from build123d import *

# Parameters (mm, degrees)
F0_R     = 152.4
F0_R_2   = 30.734
F1_DEPTH = 12.954
F2_R     = 165.1
F3_DEPTH = 17.78
F4_R     = 165.1
F5_DEPTH = 17.78
F6_R     = 30.1625
F7_DEPTH = 62.66538


with BuildPart() as f1:
    # F0 (on Top) → F1 (new body)
    with BuildSketch(Plane.XY):
        Circle(F0_R)
        Circle(F0_R_2, mode=Mode.SUBTRACT)
    extrude(amount=F1_DEPTH)

    # F2 (on face) → F3 (join)
    with BuildSketch(Plane(origin=(0, 0, 0), x_dir=(1, 0, 0), z_dir=(0, 0, -1))):
        Circle(F2_R)
    extrude(amount=F3_DEPTH)

    # F4 (on face) → F5 (join)
    with BuildSketch(Plane.XY.offset(12.954)):
        Circle(F4_R)
    extrude(amount=F5_DEPTH)

    # F6 (on face) → F7 (cut)
    with BuildSketch(Plane(origin=(0, 0, -17.78), x_dir=(1, 0, 0), z_dir=(0, 0, -1))):
        Circle(F6_R)
    extrude(amount=-F7_DEPTH, mode=Mode.SUBTRACT)


solid = f1.part
Model file for the job. Use its own axes, mm. A direction names the side the tool comes from. Coordinates: 2 decimals unless noted, no trailing zeros. Write each loop counter-clockwise with the first axis right and the second up, starting at its lowest first coordinate (ties: lowest second). Pieces come first, ordered by that corner, then holes. Notation, with made-up numbers: (-25.75, 12.5) -> (6.25, 12.5) arc R23 cw to (6.25, 37.5) -> close; hole circle Ø3 at (71.5, -17). An arc over 180 degrees is marked (long way). One line per item, written item: value. Start each with the question number.
1) Which spindle directions (+Z, -Z, +X, -X, +Y, -Y) get a long thin tool onto all of the face, cutting with end or side? Do faces 4 (the face through (-35.79, -161.174, 21.72)), 5 (the face through (48, -146, 12.954)). Say none if no direction does.
2) Slice it at D-D on z = 18. Write the cut outline in (x, y) (1 decimal).
3) Probe probe 1 along X at (y, z) = (0, -11.75); probe 2 along Y at (x, z) = (0, 7.75). List the from-to ranges inside material, lowest first.
4) Slice it at C-C on x = 45.5. Write the cut outline in (y, z), then the cut area to 3 significant figures.
5) Pull direction X, two halves, no side cores. Call faces 1 (the face through (48, 146, 0)), 2 (the face through (-120.94, -92.73, 6.39)), 3 (the face through (23, 20, 0)): +X half, -X half, draft (parallel to the pull), parting line (faces both ways), or undercut.
6) Flat gauge pins, fed straight in: pin 1 Ø12 at (y, z) = (-114.5, -11) entering from -X; pin 2 Ø5 at (y, z) = (78.5, 17) entering from -X; pin 3 Ø10 at (y, z) = (-96, 25) entering from +X; pin 4 Ø18.5 at (x, y) = (13.5, 8) entering from +Z. Where does each tip first touch, or does it go through?
7) Slice it at A-A on y = 0. Write the cut outline in (x, z), then the cut area to 3 significant figures.
Answers follow:
1. face 4: +Z, -Z
1. face 5: none
2. outline: circle Ø330.2 at (0, 0); hole circle Ø60.3 at (0, 0)
3. probe 1: -165.1 to -30.16, 30.16 to 165.1
3. probe 2: -152.4 to -30.73, 30.73 to 152.4
4. outline: (-158.71, -17.78) -> (158.71, -17.78) -> (158.71, 0) -> (145.45, 0) -> (145.45, 12.95) -> (158.71, 12.95) -> (158.71, 30.73) -> (-158.71, 30.73) -> (-158.71, 12.95) -> (-145.45, 12.95) -> (-145.45, 0) -> (-158.71, 0) -> close
4. area: 15,100 mm2
5. face 1: draft
5. face 2: parting line
5. face 3: undercut
6. pin 1: x = -124.44
6. pin 2: x = -146.57
6. pin 3: x = 137.76
6. pin 4: through
7. outline: (-165.1, -17.78) -> (-30.16, -17.78) -> (-30.16, 0) -> (-30.73, 0) -> (-30.73, 12.95) -> (-30.16, 12.95) -> (-30.16, 30.73) -> (-165.1, 30.73) -> (-165.1, 12.95) -> (-152.4, 12.95) -> (-152.4, 0) -> (-165.1, 0) -> close; (30.16, -17.78) -> (165.1, -17.78) -> (165.1, 0) -> (152.4, 0) -> (152.4, 12.95) -> (165.1, 12.95) -> (165.1, 30.73) -> (30.16, 30.73) -> (30.16, 12.95) -> (30.73, 12.95) -> (30.73, 0) -> (30.16, 0) -> close
7. area: 12,700 mm2
